```python
from build123d import *

# Parameters (mm, degrees)
F2_SIZE = 1.5
F3_R    = 2


with BuildPart() as f1:
    # F0 (on Right) → F1 (revolve)
    with BuildSketch(Plane.YZ):
        Polygon((-3.958115, 0), (17.041885, 0), (17.041885, 5), (11.041885, 5), (11.041885, 3), (-3.958115, 3), align=None)
    revolve(axis=Axis((0, 6.541885, 0), (0, 1, 0)))

    # F2
    f2_edges = [f1.edges().sort_by_distance(p)[0] for p in [
        (0, -3.958115, -3),
    ]]
    chamfer(f2_edges, length=F2_SIZE)

    # F3
    f3_edges = [f1.edges().sort_by_distance(p)[0] for p in [
        (0, 17.041885, -5),
    ]]
    fillet(f3_edges, radius=F3_R)


solid = f1.part
```
Here's how the part is built. I have some questions about the finished solid (model axes, mm). A direction names the side the tool comes from. Give positions to 0.01 mm unless a question says otherwise; leave off trailing zeros. Order: outer loops, then holes, each group sorted by start corner. A loop starts at its lowest first (then second) coordinate and runs counter-clockwise, first axis right, second up. Notation, with made-up numbers: M 22.5,49.5 L 67.5,49.5 A28 ccw 67.5,68.5 Z; hole C 39,55 d10. An arc over 180 degrees is marked long. Use a Markdown table: item, result. Add a question column.
1. For pin 1 Ø3 at (x, z) = (-0.5, 3.5) entering from +Y; pin 2 Ø5 at (x, y) = (-3, 3.5) entering from +Z; pin 3 Ø1.5 at (x, y) = (1.5, 8.5) entering from +Z; pin 4 Ø1.5 at (x, z) = (-3.5, 3) entering from +Y, each with a flat end and sliding along its axis, tell me the tip position at first contact or that it passes through.
2. Suppose I cut it at A-A (z = 0). List the corners of the cut face in (x, y) for me.
3. Suppose I cut it at B-B (x = 0). List the corners of the cut face in (y, z) for me, and give its area (3 significant figures).
4. I need wall thicknesses on probe 1 along Y at (x, z) = (-0.5, 3); probe 2 along X at (y, z) = (7, 0); probe 3 along Z at (x, y) = (2, 15.5). Which ranges of each line are inside material? Lowest first, please. Write a range as from..to.
5. On a 3-axis mill with a long thin cutter (end or side, diameter ignored), from which of +Z, -Z, +X, -X, +Y, -Y can I reach the whole of each face in a straight line? I mean faces 1 (the flat face through (0, -3.958, 0)), 2 (the flat face through (0.1, 11.042, 3.3)). Say none if no direction works.
6. Suppose I cut it at C-C (y = 1.5). List the corners of the cut face in (x, z) for me.
Results list:
| question | item | result |
|---|---|---|
| 1 | pin 1 | stops at y = 17.04 |
| 1 | pin 2 | stops at z = 2.96 |
| 1 | pin 3 | stops at z = 2.9 |
| 1 | pin 4 | stops at y = 16.85 |
| 2 | outline | M -5,11.04 L -3,11.04 L -3,-2.46 L -1.5,-3.96 L 1.5,-3.96 L 3,-2.46 L 3,11.04 L 5,11.04 L 5,15.04 A2 ccw 3,17.04 L -3,17.04 A2 ccw -5,15.04 Z |
| 3 | outline | M -3.96,-1.5 L -2.46,-3 L 11.04,-3 L 11.04,-5 L 15.04,-5 A2 ccw 17.04,-3 L 17.04,3 A2 ccw 15.04,5 L 11.04,5 L 11.04,3 L -2.46,3 L -3.96,1.5 Z |
| 3 | area | 146 mm² |
| 4 | probe 1 | y = 11.04..17.04 |
| 4 | probe 2 | x = -3..3 |
| 4 | probe 3 | z = -4.52..4.52 |
| 5 | face 1 | +Z, -Z, +X, -X, -Y |
| 5 | face 2 | -Y |
| 6 | outline | C 0,0 d6 |
